```python
from build123d import *

# Parameters (mm, degrees)
SKETCH1_W           = 38.1
SKETCH1_H           = 38.1
SKETCH1_R           = 3.175
BOSS_EXTRUDE1_DEPTH = 1.984375
SKETCH2_W           = 38.1
SKETCH2_H           = 36.115625
SKETCH2_R           = 3.175
BOSS_EXTRUDE2_DEPTH = 1.984375


with BuildPart() as part:
    # Sketch1 → Boss-Extrude1 (new body)
    with BuildSketch(Plane(origin=(0, 0, 0), x_dir=(1, 0, 0), z_dir=(0, 1, 0))):
        with Locations((19.05, -19.05)):
            Rectangle(SKETCH1_W, SKETCH1_H)
        with Locations(Location((19.05, -30.48, 0), (0, 0, 270))):
            Circle(SKETCH1_R, mode=Mode.SUBTRACT)
        with Locations(Location((8.89, -20.955, 0), (0, 0, 270))):
            Circle(SKETCH1_R, mode=Mode.SUBTRACT)
        with Locations(Location((29.21, -17.78, 0), (0, 0, 270))):
            Circle(SKETCH1_R, mode=Mode.SUBTRACT)
    extrude(amount=BOSS_EXTRUDE1_DEPTH)

    # Sketch2 → Boss-Extrude2 (add)
    with BuildSketch(Plane.XY):
        with Locations((19.05, 20.0421875)):
            Rectangle(SKETCH2_W, SKETCH2_H)
        with Locations((19.05, 30.48)):
            Circle(SKETCH2_R, mode=Mode.SUBTRACT)
        with Locations((8.89, 17.78)):
            Circle(SKETCH2_R, mode=Mode.SUBTRACT)
        with Locations((29.21, 20.955)):
            Circle(SKETCH2_R, mode=Mode.SUBTRACT)
    extrude(amount=BOSS_EXTRUDE2_DEPTH)


solid = part.part
```
Work out the finished part from the listing and answer in its coordinate system (mm). A direction names the side the tool comes from. Coordinates: 2 decimals unless noted, no trailing zeros. Write each loop counter-clockwise with the first axis right and the second up, starting at its lowest first coordinate (ties: lowest second). Pieces come first, ordered by that corner, then holes.
Q1. A cutting plane is placed at B-B, the plane x = 29.21. Give the vertices of the cut face in (y, z) (3 decimals), then the cut area to 3 significant figures.
Q2. Determine the mould class of faces 3 (the face through (32.24, 21.91, 0.98)), 4 (the face through (19, 38.1, 1)), 5 (the face through (38.1, 10, 1)) for opening direction X: released by +X, released by -X, zero draft, split by the parting line, or undercut.
Q3. A cutting plane is placed at A-A, the plane y = 30.48. Give the vertices of the cut face in (x, z) (3 decimals), then the cut area to 3 significant figures.
Q4. Find the intervals of material crossed by line 1 (Z direction, x = 23.5, y = 11.5), in increasing order.
Q5. Each of these flat-tipped pins is pushed along its axis until it touches: pin 1 Ø5 at (x, z) = (25.5, 30.5) entering from -Y; pin 2 Ø5.5 at (x, z) = (8.89, 20.955) entering from -Y; pin 3 Ø4 at (x, z) = (28.5, 10) entering from +Y; pin 4 Ø7.5 at (x, y) = (29.21, 20.955) entering from +Z. Where does it stop, or does it pass through?
Q6. A cutting plane is placed at D-D, the plane y = 19. Give the vertices of the cut face in (x, z).
Q7. Which of the six approach directions +Z, -Z, +X, -X, +Y, -Y give full straight-line access (tool end or side, diameter ignored) to faces 1 (the face through (16.53, 28.55, 0.98)), 2 (the face through (19, 20, 1.984))?
Findings below:
1. outline: (0, 0) - (17.78, 0) - (17.78, 1.984) - (1.984, 1.984) - (1.984, 14.605) - (0, 14.605) - close; (0, 20.955) - (1.984, 20.955) - (1.984, 38.1) - (0, 38.1) - close; (24.13, 0) - (38.1, 0) - (38.1, 1.984) - (24.13, 1.984) - close
1. area: 122 mm2
2. face 3: undercut
2. face 4: zero draft
2. face 5: released by +X
3. outline: (0, 0) - (15.875, 0) - (15.875, 1.984) - (0, 1.984) - close; (22.225, 0) - (38.1, 0) - (38.1, 1.984) - (22.225, 1.984) - close
3. area: 63.0 mm2
4. line 1: z = 0 to 1.98
5. pin 1: stops at y = 0
5. pin 2: passes through
5. pin 3: stops at y = 1.98
5. pin 4: stops at z = 1.98
6. outline: (0, 0) - (5.96, 0) - (5.96, 1.98) - (0, 1.98) - close; (11.82, 0) - (26.71, 0) - (26.71, 1.98) - (11.82, 1.98) - close; (31.71, 0) - (38.1, 0) - (38.1, 1.98) - (31.71, 1.98) - close
7. face 1: +Z, -Z
7. face 2: +Z, +X, -X, +Y
